```python
from build123d import *

# Parameters (mm, degrees)
SKETCH1_W                      = 50
SKETCH1_H                      = 42.1
SKETCH1_W_2                    = 30
SKETCH1_H_2                    = 22.1
BOSS_EXTRUDE2_DEPTH            = 3
FILLET1_R                      = 1
SKETCH2_W                      = 50
SKETCH2_H                      = 42.1
SKETCH2_W_2                    = 40
SKETCH2_H_2                    = 32.1
BOSS_EXTRUDE3_DEPTH            = 17
SKETCH3_W                      = 25
SKETCH3_H                      = 20
BOSS_EXTRUDE4_DEPTH            = 5
M4_CLEARANCE_HOLE1_D           = 4.5
M4_CLEARANCE_HOLE1_CSINK_D     = 4.55
M4_CLEARANCE_HOLE1_CSINK_ANGLE = 90
FILLET2_R                      = 12


with BuildPart() as part:
    # Sketch1 → Boss-Extrude2 (new body)
    with BuildSketch(Plane(origin=(0, 0, 0), x_dir=(1, 0, 0), z_dir=(0, 1, 0))):
        Rectangle(SKETCH1_W, SKETCH1_H)
        Rectangle(SKETCH1_W_2, SKETCH1_H_2, mode=Mode.SUBTRACT)
    extrude(amount=-BOSS_EXTRUDE2_DEPTH)

    # Fillet1
    fillet1_edges = [part.edges().sort_by_distance(p)[0] for p in [
        (15, 0, 0),
        (0, 0, -11.05),
        (-15, 0, 0),
        (0, 0, 11.05),
    ]]
    fillet(fillet1_edges, radius=FILLET1_R)

    # Sketch2 → Boss-Extrude3 (add)
    with BuildSketch(Plane.XZ.offset(3)):
        Rectangle(SKETCH2_W, SKETCH2_H)
        Rectangle(SKETCH2_W_2, SKETCH2_H_2, mode=Mode.SUBTRACT)
    extrude(amount=BOSS_EXTRUDE3_DEPTH)

    # Sketch3 → Boss-Extrude4 (add)
    with BuildSketch(Plane(origin=(0, 0, -21.05), x_dir=(-1, 0, 0), z_dir=(0, 0, -1))):
        with Locations((-37.5, -10)):
            Rectangle(SKETCH3_W, SKETCH3_H)
    boss_extrude4 = extrude(amount=-BOSS_EXTRUDE4_DEPTH)

    # M4 Clearance Hole1 (through all)
    with Locations(Plane(origin=(43, -10, -21.05), x_dir=(-1, 0, 0), z_dir=(0, 0, -1))):
        with Locations((0, 0)):
            m4_clearance_hole1 = CounterSinkHole(M4_CLEARANCE_HOLE1_D / 2, M4_CLEARANCE_HOLE1_CSINK_D / 2, counter_sink_angle=M4_CLEARANCE_HOLE1_CSINK_ANGLE)

    # Mirror4: Boss-Extrude4, M4 Clearance Hole1 across plane
    add(boss_extrude4.mirror(Plane(origin=(0, 0, 0), x_dir=(0, 0, 1), z_dir=(1, 0, 0))))
    add(m4_clearance_hole1.mirror(Plane(origin=(0, 0, 0), x_dir=(0, 0, 1), z_dir=(1, 0, 0))), mode=Mode.SUBTRACT)

    # Fillet2
    fillet2_edges = [part.edges().sort_by_distance(p)[0] for p in [
        (25, -10, -16.05),
        (-25, -10, -16.05),
    ]]
    fillet(fillet2_edges, radius=FILLET2_R)


solid = part.part
```
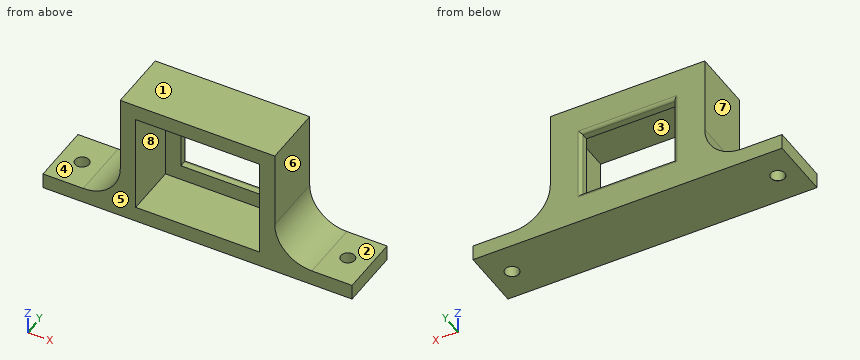
Work out the finished part from the listing and answer in its coordinate system (mm). Face numbers are marked on the shaded views. A direction names the side the tool comes from. Coordinates: 2 decimals unless noted, no trailing zeros. Order: outer loops, then holes, each group sorted by start corner. A loop starts at its lowest first (then second) coordinate and runs counter-clockwise, first axis right, second up. Notation, with made-up numbers: (27.25, 61.5) - (31.25, 61.5) arc R21 cw to (31.25, 70.5) - close; hole circle Ø3 at (64.25, 28). An arc over 180 degrees is marked (long way). Answer as a JSON object with one key per item and string values.
1. Find section C-C on z = 6. Determine the outline of the cut face in (x, y), plus the area to 3 significant figures.
Output values:
{"outline": "(-25, -20) - (-20, -20) - (-20, -3) - (-15, -3) - (-15, -1) arc R1 ccw to (-16, 0) - (-25, 0) - close; (15, -3) - (20, -3) - (20, -20) - (25, -20) - (25, 0) - (16, 0) arc R1 ccw to (15, -1) - close", "area": "230 mm²"}
2. Find section D-D on y = -5.5. Determine the outline of the cut face in (x, z), plus the area to 3 significant figures.
Output values:
{"outline": "(-50, -21.05) - (50, -21.05) - (50, -16.05) - (37, -16.05) arc R12 cw to (25, -4.05) - (25, 21.05) - (-25, 21.05) - (-25, -4.05) arc R12 cw to (-37, -16.05) - (-50, -16.05) - close; hole (-20, -16.05) - (20, -16.05) - (20, 16.05) - (-20, 16.05) - close", "area": "1,130 mm²"}
3. Consider line 1 (X direction, y = -10, z = -17.8); line 2 (X direction, y = -8.25, z = 4.5); line 3 (Y direction, x = -43, z = -17.6). Determine where each line is inside the solid, lowest interval first.
Output values:
{"line 1": "x = -50 to -45.25, -40.75 to 40.75, 45.25 to 50", "line 2": "x = -25 to -20, 20 to 25", "line 3": "y = -20 to -12.25, -7.75 to 0"}
4. Find section B-B on x = 14. Determine the outline of the cut face in (y, z), plus the area to 3 significant figures.
Output values:
{"outline": "(-20, -21.05) - (0, -21.05) - (0, -12.05) arc R1 ccw to (-1, -11.05) - (-3, -11.05) - (-3, -16.05) - (-20, -16.05) - close; (-20, 16.05) - (-3, 16.05) - (-3, 11.05) - (-1, 11.05) arc R1 ccw to (0, 12.05) - (0, 21.05) - (-20, 21.05) - close", "area": "230 mm²"}
5. The mould has two halves that part along X. Classify the marked faces 6, 7 and 8: +X half, -X half, draft (parallel to the pull), parting line (faces both ways), or undercut.
Output values:
{"face 6": "+X half", "face 7": "-X half", "face 8": "undercut"}
6. Find section A-A on y = -10. Determine the outline of the cut face in (x, z) (3 decimals).
Output values:
{"outline": "(-50, -21.05) - (-45.275, -21.05) - (-45.25, -21.025) - (-45.25, -16.05) - (-50, -16.05) - close; (-40.75, -21.025) - (-40.725, -21.05) - (40.725, -21.05) - (40.75, -21.025) - (40.75, -16.05) - (37, -16.05) arc R12 cw to (25, -4.05) - (25, 21.05) - (-25, 21.05) - (-25, -4.05) arc R12 cw to (-37, -16.05) - (-40.75, -16.05) - close; (45.25, -21.025) - (45.275, -21.05) - (50, -21.05) - (50, -16.05) - (45.25, -16.05) - close; hole (-20, -16.05) - (20, -16.05) - (20, 16.05) - (-20, 16.05) - close"}
7. A tool of negligible diameter and unlimited length cuts with its end or side. For the marked faces 1, 2, 3, 4 and 5, from which of +Z, -Z, +X, -X, +Y, -Y can it reach the whole face along a straight path? Write none if from no direction.
Output values:
{"face 1": "+Z, +X, -X, +Y, -Y", "face 2": "+Z, +X, +Y, -Y", "face 3": "-Y", "face 4": "+Z, -X, +Y, -Y", "face 5": "+Z, -Z, +X, -X, -Y"}
8. Each of these flat-tipped pins is pushed along its axis until it touches: P1, Ø10, axis at y = -7, z = 6, coming from the +X side; P2, Ø4, axis at x = 43, y = -14.5, coming from the +Z side; P3, Ø2, axis at x = -34.5, y = -18, coming from the +Z side. Where does it stop, or does it pass through?
Output values:
{"P1": "stops at x = 25", "P2": "stops at z = -16.05", "P3": "stops at z = -15.53"}
